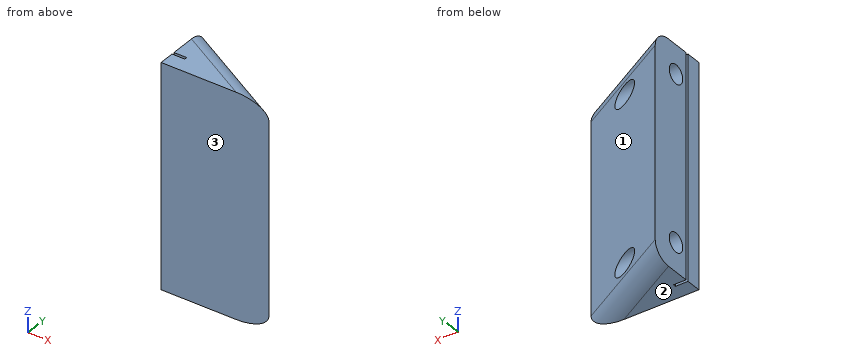
from build123d import *

# Parameters (mm, degrees)
BOSS_EXTRUDE1_DEPTH = 261.62
SKETCH3_R           = 11.049
SKETCH3_R_2         = 11.103550021
CUT_EXTRUDE2_DEPTH  = 109.728
SKETCH2_W           = 14.986
SKETCH2_H           = 3.124293054
CUT_EXTRUDE3_DEPTH  = 268.224
VARFILLET1_START    = -36
VARFILLET1_DEPTH    = 148


with BuildPart() as part:
    # Sketch1 → Boss-Extrude1 (new body)
    with BuildSketch(Plane.XY):
        Polygon((0, 0), (0, 71.882), (127, 0), align=None)
    extrude(amount=BOSS_EXTRUDE1_DEPTH)

    # Sketch3 → Cut-Extrude2 (cut)
    with BuildSketch(Plane.ZY):
        with Locations((227.711, 37.719)):
            Circle(SKETCH3_R)
        with Locations((34.001176145, 37.719)):
            Circle(SKETCH3_R_2)
    extrude(amount=-CUT_EXTRUDE2_DEPTH, mode=Mode.SUBTRACT)

    # Sketch2 → Cut-Extrude3 (cut)
    with BuildSketch(Plane.XY.offset(261.62)):
        with Locations((7.493, 19.538461467)):
            Rectangle(SKETCH2_W, SKETCH2_H)
    extrude(amount=-CUT_EXTRUDE3_DEPTH, mode=Mode.SUBTRACT)

    # VarFillet1: read off the stored shape, not the designer's step
    # VarFillet1 outline → VarFillet1 (cut)
    with BuildSketch(Plane(origin=(0, 0, 0), x_dir=(0.4925733480628631, 0.8702709329732561, 0), z_dir=(0.8702709329732561, -0.49257334806286307, 0)).offset(VARFILLET1_START)):
        with BuildLine():
            Line((62.556815204, 0), (62.556815204, 19.05))
            ThreePointArc((62.556815204, 19.05), (56.977199386, 5.579615818), (43.506815204, 0))
            Line((43.506815204, 0), (62.556815204, 0))
        make_face()
        with BuildLine():
            ThreePointArc((43.506815204, 261.62), (56.977199386, 256.040384182), (62.556815204, 242.57))
            Line((62.556815204, 242.57), (62.556815204, 261.62))
            Line((62.556815204, 261.62), (43.506815204, 261.62))
        make_face()
    extrude(amount=VARFILLET1_DEPTH, mode=Mode.SUBTRACT)


solid = part.part
Model file for the job. Use its own axes, mm. Face numbers are marked on the shaded views. Coordinates: 2 decimals unless noted, no trailing zeros. Order: outer loops, then holes, each group sorted by start corner. A loop starts at its lowest first (then second) coordinate and runs counter-clockwise, first axis right, second up. Notation, with made-up numbers: M 86.25,69 L 93.25,69 A29 ccw 93.25,108 Z; hole C 74.25,-10.5 d8. An arc over 180 degrees is marked long. Return JSON: item names as keys, results as strings.
1. Saw through at C-C (y = 46). Give the number of separate pieces and of enclosed holes in the cut face, and give its area (3 significant figures).
Ans:
{"separate pieces": "3", "enclosed holes": "0", "area": "10,300 mm^2"}
2. Pull direction Y, two halves, no side cores. Call the marked faces 1, 2 and 3: +Y half, -Y half, draft (parallel to the pull), parting line (faces both ways), or undercut.
Ans:
{"face 1": "+Y half", "face 2": "draft", "face 3": "-Y half"}
3. Flat gauge pins, fed straight in: pin 1 (3 mm diameter, centred on y = 52, z = 50.5, fed in from +X); pin 2 (1.5 mm diameter, centred on x = 48, y = 43, fed in from -Z); pin 3 (12 mm diameter, centred on x = 103.5, z = 124.5, fed in from +Y). Where does each tip first touch, or does it go through?
Ans:
{"pin 1": "x = 37.78", "pin 2": "z = 10.08", "pin 3": "y = 16.7"}
4. Drill centre lines: probe 1 along Z at (x, y) = (53, 34); probe 2 along Y at (x, z) = (42, 115); probe 3 along X at (y, z) = (60, 212). Where is each one in solid material? Low to high.
Ans:
{"probe 1": "4.41 to 23.54, 44.46 to 217.31, 238.12 to 257.21", "probe 2": "0 to 48.11", "probe 3": "0 to 20.99"}
5. Saw through at B-B (z = 81). Give the cut face in (x, y).
Ans:
{"outline": "M 0,0 L 127,0 L 0,71.88 L 0,21.1 L 14.99,21.1 L 14.99,17.98 L 0,17.98 Z"}
6. Saw through at A-A (z = 26). Give the cut face in (x, y), and give its area (3 significant figures).
Ans:
{"outline": "M 0,0 L 127,0 L 73.96,30.02 L 0,30.02 L 0,21.1 L 14.99,21.1 L 14.99,17.98 L 0,17.98 Z; M 0,45.42 L 46.76,45.42 L 0,71.88 Z", "area": "3,590 mm^2"}
